Can you work these out from the model? Positions are in its coordinate system, mm. Face numbers are marked on the shaded views. A direction names the side the tool comes from. Give positions to 0.01 mm unless a question says otherwise; leave off trailing zeros. Loops run counter-clockwise (first coordinate to the right, second up) from the corner with the lowest first, then second, coordinate; pieces in that order, holes last. Notation, with made-up numbers: (-4, 0.5) -> (52, 0.5) arc R14 cw to (52, 4.5) -> close; hole circle Ø10 at (53, -34). An arc over 180 degrees is marked (long way). Use CSV: the item, a comma, the result in double quotes.
from build123d import *

# Parameters (mm, degrees)
SKETCH_3_R          = 23.35
EXTRUDE_3_DEPTH     = 6.4
SKETCH_2_R          = 21.8
CUT_EXTRUDE_1_DEPTH = 1.63
CUT_EXTRUDE_START   = 1.63
CUT_EXTRUDE_2_DEPTH = 2.6
SKETCH_5_R          = 1.35000002
SKETCH_5_R_2        = 1.35
CUT_EXTRUDE_3_DEPTH = 4.77
CUT_EXTRUDE_START_2 = 4.23
SKETCH_5_3_R        = 5.5
CUT_EXTRUDE_4_DEPTH = 2.17
CHAMFER_1_SIZE      = 0.75
CUT_EXTRUDE_START_3 = 6.4
SKETCH_6_R          = 2.6
CUT_EXTRUDE_5_DEPTH = 1
CHAMFER_2_SIZE      = 1.29
CHAMFER_2_SIZE_2    = 2.385
CHAMFER_3_SIZE      = 0.25
CHAMFER_4_SIZE      = 0.8
CUT_EXTRUDE_7_DEPTH = 0.4
CUT_EXTRUDE_8_DEPTH = 1.5


with BuildPart() as part:
    # 草图3 → 凸台-拉伸3 (new body)
    with BuildSketch(Plane.XY):
        with Locations((100.00000066, 100.00000066)):
            Circle(SKETCH_3_R)
    extrude(amount=EXTRUDE_3_DEPTH)

    # 草图2 → 切除-拉伸1 (cut)
    with BuildSketch(Plane.XY):
        with Locations((100.00000066, 100.00000066)):
            Circle(SKETCH_2_R)
    extrude(amount=CUT_EXTRUDE_1_DEPTH, mode=Mode.SUBTRACT)

    # 草图4 → 切除-拉伸2 (cut)
    with BuildSketch(Plane.XY.offset(CUT_EXTRUDE_START)):
        with BuildLine():
            Line((98.171, 114.173), (98.171, 115.57))
            ThreePointArc((98.171, 115.57), (98.282592316, 115.839407684), (98.552, 115.951))
            Line((98.552, 115.951), (102.87, 115.951))
            ThreePointArc((102.87, 115.951), (103.139407684, 115.839407684), (103.251, 115.57))
            Line((103.251, 115.57), (103.251, 114.808))
            ThreePointArc((103.251, 114.808), (103.362592316, 114.538592316), (103.632, 114.427))
            Line((103.632, 114.427), (109.728, 114.427))
            ThreePointArc((109.728, 114.427), (110.44642049, 114.12942049), (110.744, 113.411))
            Line((110.744, 113.411), (110.744, 110.363))
            ThreePointArc((110.744, 110.363), (110.892789755, 110.003789755), (111.252, 109.855))
            Line((111.252, 109.855), (115.951, 109.855))
            ThreePointArc((115.951, 109.855), (116.489815367, 109.631815367), (116.713, 109.093))
            Line((116.713, 109.093), (116.713, 104.521))
            ThreePointArc((116.713, 104.521), (117.01057951, 103.80257951), (117.729, 103.505))
            ThreePointArc((117.729, 103.505), (118.088210245, 103.356210245), (118.237, 102.997))
            Line((118.237, 102.997), (118.237, 102.362))
            ThreePointArc((118.237, 102.362), (118.162605122, 102.182394878), (117.983, 102.108))
            Line((117.983, 102.108), (116.586, 102.108))
            ThreePointArc((116.586, 102.108), (116.226789755, 102.256789755), (116.078, 102.616))
            ThreePointArc((116.078, 102.616), (115.892012806, 103.065012806), (115.443, 103.251))
            Line((115.443, 103.251), (106.426, 103.251))
            ThreePointArc((106.426, 103.251), (105.976987194, 103.065012806), (105.791, 102.616))
            Line((105.791, 102.616), (105.791, 95.377))
            ThreePointArc((105.791, 95.377), (105.939789755, 95.017789755), (106.299, 94.869))
            Line((106.299, 94.869), (115.57, 94.869))
            ThreePointArc((115.57, 94.869), (115.749605122, 94.794605122), (115.824, 94.615))
            Line((115.824, 94.615), (115.824, 92.202))
            ThreePointArc((115.824, 92.202), (115.638012806, 91.752987194), (115.189, 91.567))
            Line((115.189, 91.567), (115.062, 91.567))
            ThreePointArc((115.062, 91.567), (114.702789755, 91.418210245), (114.554, 91.059))
            Line((114.554, 91.059), (114.554, 89.662))
            ThreePointArc((114.554, 89.662), (114.405210245, 89.302789755), (114.046, 89.154))
            Line((114.046, 89.154), (111.887, 89.154))
            ThreePointArc((111.887, 89.154), (111.527789755, 89.005210245), (111.379, 88.646))
            Line((111.379, 88.646), (111.379, 87.884))
            ThreePointArc((111.379, 87.884), (111.230210245, 87.524789755), (110.871, 87.376))
            Line((110.871, 87.376), (109.855, 87.376))
            ThreePointArc((109.855, 87.376), (109.495789755, 87.227210245), (109.347, 86.868))
            Line((109.347, 86.868), (109.347, 85.344))
            ThreePointArc((109.347, 85.344), (109.161012806, 84.894987194), (108.712, 84.709))
            Line((108.712, 84.709), (107.188, 84.709))
            ThreePointArc((107.188, 84.709), (107.008394878, 84.634605122), (106.934, 84.455))
            ThreePointArc((106.934, 84.455), (106.896802561, 84.365197439), (106.807, 84.328))
            Line((106.807, 84.328), (103.759, 84.328))
            ThreePointArc((103.759, 84.328), (103.130382072, 84.067617928), (102.87, 83.439))
            ThreePointArc((102.87, 83.439), (102.758407684, 83.169592316), (102.489, 83.058))
            Line((102.489, 83.058), (96.901, 83.058))
            ThreePointArc((96.901, 83.058), (96.451987194, 83.243987194), (96.266, 83.693))
            Line((96.266, 83.693), (96.266, 94.869))
            ThreePointArc((96.266, 94.869), (95.931223051, 95.677223051), (95.123, 96.012))
            ThreePointArc((95.123, 96.012), (94.314776949, 96.346776949), (93.98, 97.155))
            Line((93.98, 97.155), (93.98, 103.632))
            ThreePointArc((93.98, 103.632), (94.351974388, 104.530025612), (95.25, 104.902))
            ThreePointArc((95.25, 104.902), (96.058223051, 105.236776949), (96.393, 106.045))
            Line((96.393, 106.045), (96.393, 113.665))
            ThreePointArc((96.393, 113.665), (96.541789755, 114.024210245), (96.901, 114.173))
            Line((96.901, 114.173), (98.171, 114.173))
        make_face()
    extrude(amount=CUT_EXTRUDE_2_DEPTH, mode=Mode.SUBTRACT)

    # 草图5 → 切除-拉伸3 (cut)
    with BuildSketch(Plane.XY.offset(CUT_EXTRUDE_START)):
        with Locations((113.72499988, 100.00000066)):
            Circle(SKETCH_5_R)
        with Locations((93.13749978, 111.8861999)):
            Circle(SKETCH_5_R_2)
        with Locations((93.13750232, 88.11380142)):
            Circle(SKETCH_5_R)
    extrude(amount=CUT_EXTRUDE_3_DEPTH, mode=Mode.SUBTRACT)

    # 草图5<3> → 切除-拉伸4 (cut)
    with BuildSketch(Plane.XY.offset(CUT_EXTRUDE_START_2)):
        with Locations((100.00000066, 100.00000066)):
            Circle(SKETCH_5_3_R)
    extrude(amount=CUT_EXTRUDE_4_DEPTH, mode=Mode.SUBTRACT)

    # 倒角1
    chamfer_1_edges = [part.edges().sort_by_distance(p)[0] for p in [
        (76.65000066, 100.00000066, 6.4),
    ]]
    chamfer(chamfer_1_edges, length=CHAMFER_1_SIZE)

    # 草图6 → 切除-拉伸5 (cut)
    with BuildSketch(Plane.XY.offset(CUT_EXTRUDE_START_3)):
        with Locations((93.13749978, 111.8861999)):
            Circle(SKETCH_6_R)
        with Locations((93.13750232, 88.11380142)):
            Circle(SKETCH_6_R)
        with Locations((113.72499988, 100.00000066)):
            Circle(SKETCH_6_R)
    extrude(amount=-CUT_EXTRUDE_5_DEPTH, mode=Mode.SUBTRACT)

    # 倒角2
    # the kernel refuses this chamfer: 2.385, 1.29 mm, written as the material it takes off along each edge
    with BuildSketch(Plane(origin=(113.72499988, 100.00000066, 5.4), x_dir=(1, 0, 0), z_dir=(0, 1, 0))) as chamfer_2_piece_1_section:
        Polygon((1.35000002 + CHAMFER_2_SIZE, 0), (1.35000002, CHAMFER_2_SIZE_2), (1.35000002, 0), align=None)
    chamfer_2_piece_1 = revolve(axis=Axis((113.72499988, 100.00000066, 5.4), (0, 0, -1)), mode=Mode.PRIVATE)
    chamfer_2_piece_1 = chamfer_2_piece_1 & Plane(origin=(113.72499988, 100.00000066, 4.141318071), x_dir=(1, 0, 0), z_dir=(0, 0, 1)) * Cylinder(2.6, 11, mode=Mode.PRIVATE)
    add(chamfer_2_piece_1, mode=Mode.SUBTRACT)
    with BuildSketch(Plane(origin=(93.13750232, 88.11380142, 5.4), x_dir=(1, 0, 0), z_dir=(0, 1, 0))) as chamfer_2_piece_2_section:
        Polygon((1.35000002 + CHAMFER_2_SIZE, 0), (1.35000002, CHAMFER_2_SIZE_2), (1.35000002, 0), align=None)
    chamfer_2_piece_2 = revolve(axis=Axis((93.13750232, 88.11380142, 5.4), (0, 0, -1)), mode=Mode.PRIVATE)
    chamfer_2_piece_2 = chamfer_2_piece_2 & Plane(origin=(93.13750232, 88.11380142, 4.141318071), x_dir=(1, 0, 0), z_dir=(0, 0, 1)) * Cylinder(2.6, 11, mode=Mode.PRIVATE)
    add(chamfer_2_piece_2, mode=Mode.SUBTRACT)
    with BuildSketch(Plane(origin=(93.13749978, 111.8861999, 5.4), x_dir=(1, 0, 0), z_dir=(0, 1, 0))) as chamfer_2_piece_3_section:
        Polygon((1.35 + CHAMFER_2_SIZE, 0), (1.35, CHAMFER_2_SIZE_2), (1.35, 0), align=None)
    chamfer_2_piece_3 = revolve(axis=Axis((93.13749978, 111.8861999, 5.4), (0, 0, -1)), mode=Mode.PRIVATE)
    chamfer_2_piece_3 = chamfer_2_piece_3 & Plane(origin=(93.13749978, 111.8861999, 4.14131809), x_dir=(1, 0, 0), z_dir=(0, 0, 1)) * Cylinder(2.6, 11, mode=Mode.PRIVATE)
    add(chamfer_2_piece_3, mode=Mode.SUBTRACT)

    # 倒角3
    chamfer_3_edges = [part.edges().sort_by_distance(p)[0] for p in [
        (76.65000066, 100.00000066, 0),
        (78.20000066, 100.00000066, 0),
    ]]
    chamfer(chamfer_3_edges, length=CHAMFER_3_SIZE)

    # 倒角4
    chamfer_4_edges = [part.edges().sort_by_distance(p)[0] for p in [
        (94.50000066, 100.00000066, 6.4),
    ]]
    chamfer(chamfer_4_edges, length=CHAMFER_4_SIZE)

    # 草图7 → 切除-拉伸7 (cut)
    with BuildSketch(Plane.XY.offset(CUT_EXTRUDE_START_3)):
        with BuildLine():
            Line((101.153292027, 112.351983356), (100.491527321, 107.351983356))
            Line((100.491527321, 107.351983356), (98.579762615, 107.351983356))
            Line((98.579762615, 107.351983356), (97.800350851, 112.351983356))
            Line((97.800350851, 112.351983356), (99.153292027, 112.351983356))
            add(Edge.make_bspline(
                [(99.153292027, 112.351983356), (99.168921879, 112.183478907), (99.199612846, 111.852601535), (99.244769811, 111.364867467), (99.287839178, 110.894880063), (99.32934088, 110.442074285), (99.36873281, 110.007013377), (99.406549784, 109.589133158), (99.442298553, 109.189001817), (99.465495493, 108.927964622), (99.476821439, 108.800512768)],
                knots=[0, 0, 0, 0, 1.138884633, 2.23632763, 3.296435453, 4.315101947, 5.296434007, 6.236325144, 7.138882761, 8, 8, 8, 8], degree=3))
            add(Edge.make_bspline(
                [(99.476821439, 108.800512768), (99.487820182, 108.924289993), (99.50949114, 109.168169772), (99.54197814, 109.527795956), (99.57177187, 109.875936959), (99.602376256, 110.211670122), (99.631747985, 110.535509401), (99.660256803, 110.847088908), (99.687810927, 111.146723094), (99.705975255, 111.342486994), (99.714872909, 111.438380415)],
                knots=[0, 0, 0, 0, 1.126017228, 2.218605494, 3.271989625, 4.292190047, 5.273432066, 6.218480867, 7.127336737, 8, 8, 8, 8], degree=3))
            Line((99.714872909, 111.438380415), (99.800350851, 112.351983356))
            Line((99.800350851, 112.351983356), (101.153292027, 112.351983356))
        make_face()
        Polygon((101.329762615, 110.234336298), (102.447409674, 110.234336298), (102.447409674, 111.351983356), (103.212115556, 111.351983356), (103.212115556, 110.234336298), (104.329762615, 110.234336298), (104.329762615, 109.469630415), (103.212115556, 109.469630415), (103.212115556, 108.351983356), (102.447409674, 108.351983356), (102.447409674, 109.469630415), (101.329762615, 109.469630415), align=None)
    extrude(amount=-CUT_EXTRUDE_7_DEPTH, mode=Mode.SUBTRACT)

    # 草图8 → 切除-拉伸8 (cut)
    with BuildSketch(Plane.XY.offset(CUT_EXTRUDE_START)):
        Polygon((82.169, 102.87), (83.058, 102.87), (83.439, 102.489), (83.439, 98.425), (83.82, 98.044), (86.868, 98.044), (87.122, 98.298), (87.122, 101.981), (87.376, 102.235), (91.313, 102.235), (91.567, 102.489), (91.567, 107.95), (91.186, 108.331), (88.592596753, 108.331), (87.840706234, 109.082890519), (85.376287582, 109.082890519), (85.217, 108.923602937), (85.217, 108.077), (84.836, 107.696), (83.185, 107.696), (82.169, 106.68), align=None)
    extrude(amount=CUT_EXTRUDE_8_DEPTH, mode=Mode.SUBTRACT)


solid = part.part
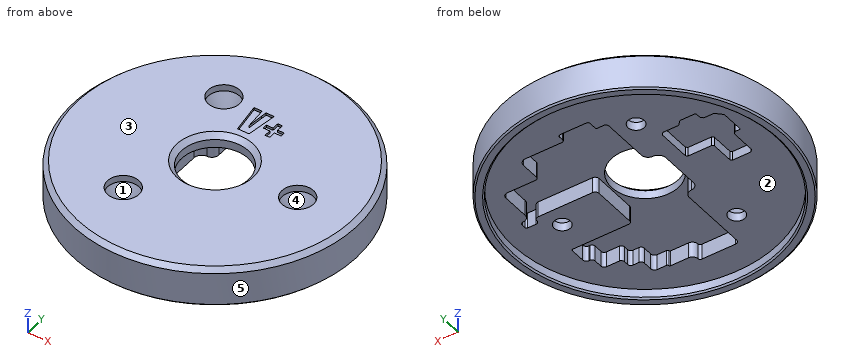
(1) If I drill on L1, parallel to Y at x = 106, z = 2.75; L2, parallel to X at y = 99, z = 5; L3, parallel to Y at x = 108, z = 3.25, over which ranges is the centre line in solid material (lowest first)? Write a range as from..to.
Answer sheet:
L1,"y = 77.43..84.33, 94.97..103.09, 114.43..122.57"
L2,"x = 76.67..94.59, 105.41..111.52, 115.93..123.33"
L3,"y = 78.06..84.71, 94.87..103.25, 114.43..121.94"
(2) Will these pins go through, and if not, where does the flat tip stop? pin 1 Ø1.5 at (y, z) = (117.5, 5.5) entering from +X; pin 2 Ø1.3 at (y, z) = (106, 2.5) entering from -X; pin 3 Ø1.6 at (y, z) = (104.5, 2.5) entering from -X (3 decimals); pin 4 Ø2.5 at (x, y) = (113.725, 100) entering from +Z.
Answer sheet:
pin 1,"stops at x = 116.27"
pin 2,"stops at x = 77.27"
pin 3,"stops at x = 76.945"
pin 4,"passes through"
(3) If we section it at A-A, the plane y = 100: Give the number of separate pieces and of enclosed holes in the cut face, then the cut area to 3 significant figures.
Answer sheet:
separate pieces,"3"
enclosed holes,"0"
area,"148 mm2"
(4) We'd pull the mould along X, two halves only. Please class the marked faces 3, 4 and 5: released by +X, released by -X, zero draft, split by the parting line, or undercut.
Answer sheet:
face 3,"zero draft"
face 4,"undercut"
face 5,"split by the parting line"
(5) If we section it at B-B, the plane z = 1: Write out the boundary of the cut face in (x, y).
Answer sheet:
outline,"circle Ø46.7 at (100, 100); hole circle Ø43.6 at (100, 100)"
(6) Which directions (+Z, -Z, +X, -X, +Y, -Y) give clear straight access to the entire face, cutting with the end or side of a thin tool? Please do the marked faces 1 and 2.
Answer sheet:
face 1,"+Z"
face 2,"-Z"
